Here's how the part is built. I have some questions about the finished solid (model axes, mm). A direction names the side the tool comes from. Round coordinates to 2 decimals unless told otherwise and drop trailing zeros. Write each loop counter-clockwise with the first axis right and the second up, starting at its lowest first coordinate (ties: lowest second). Pieces come first, ordered by that corner, then holes. Notation, with made-up numbers: M 22,44.25 L 31,44.25 A23 ccw 31,80.25 Z; hole C -7.5,89.5 d6. An arc over 180 degrees is marked long. Use a Markdown table: item, result. Add a question column.
```python
from build123d import *

# Parameters (mm, degrees)
F0_W      = 28
F0_H      = 19
F1_DEPTH  = 4
F2_W      = 20
F2_H      = 2
F3_DEPTH  = 25
F4_W      = 24
F4_H      = 2.5
F5_DEPTH  = 2
F6_W      = 2.5
F6_H      = 2
F6_H_2    = 25
F7_DEPTH  = 2
F8_W      = 2.5
F8_H      = 2
F8_H_2    = 25
F9_DEPTH  = 2
F10_W     = 28
F10_H     = 2
F11_DEPTH = 7
F12_W     = 28
F12_H     = 2
F13_DEPTH = 5
F14_W     = 28
F14_H     = 2
F15_DEPTH = 5


with BuildPart() as f1:
    # F0 (on Top) → F1 (new body)
    with BuildSketch(Plane.XY):
        with Locations((14, 9.5)):
            Rectangle(F0_W, F0_H)
    extrude(amount=F1_DEPTH)

    # F2 (on face) → F3 (join)
    with BuildSketch(Plane.XY.offset(4)):
        Polygon((0, 19), (0, 0), (4, 0), (4, 17), (4, 19), align=None)
        with Locations((14, 18)):
            Rectangle(F2_W, F2_H)
        Polygon((24, 19), (24, 17), (24, 0), (28, 0), (28, 19), align=None)
    extrude(amount=F3_DEPTH)

    # F4 (on face) → F5 (cut)
    with BuildSketch(Plane.XY.offset(4)):
        with Locations((14, 3.25)):
            Rectangle(F4_W, F4_H)
    extrude(amount=-F5_DEPTH, mode=Mode.SUBTRACT)

    # F6 (on face) → F7 (cut)
    with BuildSketch(Plane(origin=(24, 0, 0), x_dir=(0, -1, 0), z_dir=(-1, 0, 0))):
        with Locations((-3.25, 3)):
            Rectangle(F6_W, F6_H)
        with Locations((-3.25, 16.5)):
            Rectangle(F6_W, F6_H_2)
    extrude(amount=-F7_DEPTH, mode=Mode.SUBTRACT)

    # F8 (on face) → F9 (cut)
    with BuildSketch(Plane.YZ.offset(4)):
        with Locations((3.25, 3)):
            Rectangle(F8_W, F8_H)
        with Locations((3.25, 16.5)):
            Rectangle(F8_W, F8_H_2)
    extrude(amount=-F9_DEPTH, mode=Mode.SUBTRACT)

    # F10 (on face) → F11 (join)
    with BuildSketch(Plane.XY.offset(29)):
        with Locations((14, 18)):
            Rectangle(F10_W, F10_H)
    extrude(amount=F11_DEPTH)

    # F12 (on face) → F13 (join)
    with BuildSketch(Plane(origin=(0, 19, 0), x_dir=(-1, 0, 0), z_dir=(0, 1, 0))):
        with Locations((-14, 35)):
            Rectangle(F12_W, F12_H)
    extrude(amount=F13_DEPTH)

    # F14 (on face) → F15 (join)
    with BuildSketch(Plane(origin=(0, 0, 34), x_dir=(1, 0, 0), z_dir=(0, 0, -1))):
        with Locations((14, -23)):
            Rectangle(F14_W, F14_H)
    extrude(amount=F15_DEPTH)


solid = f1.part
```
Item 1: Imagine slicing it at A-A on z = 29.5. List the corners of the cut face in (x, y) for me, plus the area to 3 significant figures.
Item 2: Imagine slicing it at C-C on y = 12.5. List the corners of the cut face in (x, z) for me, plus the area to 3 significant figures.
Item 3: For pin 1 Ø0.8 at (x, y) = (9.5, 2.5) entering from +Z; pin 2 Ø5 at (x, z) = (19, 7.5) entering from -Y; pin 3 Ø10 at (x, z) = (3, 23) entering from +Y, each with a flat end and sliding along its axis, tell me the tip position at first contact or that it passes through.
Item 4: On a 3-axis mill with a long thin cutter (end or side, diameter ignored), from which of +Z, -Z, +X, -X, +Y, -Y can I reach the whole of each face in a straight line? I mean faces 1 (the face through (15.7, 4.5, 3.6)), 2 (the face through (14, 20, 34)), 3 (the face through (26, 9, 29)). Say none if no direction works.
Item 5: I need wall thicknesses on probe 1 along X at (y, z) = (3, 6); probe 2 along Y at (x, z) = (20.25, 3); probe 3 along Y at (x, z) = (21.25, 30). Which ranges of each line are inside material? Lowest first, please. Write a range as from..to.
Item 6: If we mould it in two halves opening along X, with no side actions, what happens to faces 4 (the face through (26, 3, 16)), 5 (the face through (14, 22, 32)), 6 (the face through (0, 10, 14))? For each: +X half, -X half, draft (parallel to the pull), parting line (faces both ways), or undercut.
Item 7: Imagine slicing it at B-B on x = 12.5. List the corners of the cut face in (y, z) for me, plus the area to 3 significant figures.
Item 8: Imagine slicing it at D-D on y = 2.5. List the corners of the cut face in (x, z) for me, plus the area to 3 significant figures.
The answers:
| question | item | result |
|---|---|---|
| 1 | outline | M 0,17 L 28,17 L 28,19 L 0,19 Z; M 0,22 L 28,22 L 28,24 L 0,24 Z |
| 1 | area | 112 mm² |
| 2 | outline | M 0,0 L 28,0 L 28,29 L 24,29 L 24,4 L 4,4 L 4,29 L 0,29 Z |
| 2 | area | 312 mm² |
| 3 | pin 1 | z = 2 |
| 3 | pin 2 | y = 17 |
| 3 | pin 3 | y = 19 |
| 4 | face 1 | +Z |
| 4 | face 2 | -Z, +X, -X |
| 4 | face 3 | +Z, +X, -X, -Y |
| 5 | probe 1 | 0..2, 26..28 |
| 5 | probe 2 | 0..2, 4.5..19 |
| 5 | probe 3 | 17..19, 22..24 |
| 6 | face 4 | undercut |
| 6 | face 5 | draft |
| 6 | face 6 | -X half |
| 7 | outline | M 0,0 L 19,0 L 19,34 L 22,34 L 22,29 L 24,29 L 24,36 L 17,36 L 17,4 L 4.5,4 L 4.5,2 L 2,2 L 2,4 L 0,4 Z |
| 7 | area | 155 mm² |
| 8 | outline | M 0,0 L 28,0 L 28,29 L 26,29 L 26,2 L 2,2 L 2,29 L 0,29 Z |
| 8 | area | 164 mm² |
